```python
from build123d import *

# Parameters (mm, degrees)
F0_R     = 5
F1_DEPTH = 10
F2_R     = 3
F3_DEPTH = 7
F4_W     = 0.5
F4_H     = 1
F6_SIZE  = 1
F7_SIZE  = 1


with BuildPart() as f1:
    # F0 (on Top) → F1 (new body)
    with BuildSketch(Plane.XY):
        Circle(F0_R)
    extrude(amount=F1_DEPTH)

    # F2 (on face) → F3 (join)
    with BuildSketch(Plane.XY.offset(10)):
        Circle(F2_R)
    extrude(amount=F3_DEPTH)

    # F4 (on Front) → F5 (revolve, cut)
    with BuildSketch(Plane.XZ):
        with Locations((2.75, 10.5)):
            Rectangle(F4_W, F4_H)
    revolve(axis=Axis((0, 0, 10), (0, 0, -1)), mode=Mode.SUBTRACT)

    # F6
    f6_edges = [f1.edges().sort_by_distance(p)[0] for p in [
        (-3, 0, 17),
    ]]
    chamfer(f6_edges, length=F6_SIZE)

    # F7
    f7_edges = [f1.edges().sort_by_distance(p)[0] for p in [
        (-5, 0, 0),
    ]]
    chamfer(f7_edges, length=F7_SIZE)


solid = f1.part
```
Source: CAD feature listing. Evaluate the final solid. Frame: model axes, mm. A direction names the side the tool comes from. Round coordinates to 2 decimals unless told otherwise and drop trailing zeros. Write each loop counter-clockwise with the first axis right and the second up, starting at its lowest first coordinate (ties: lowest second). Pieces come first, ordered by that corner, then holes. Notation, with made-up numbers: M 62,73.25 L 69,73.25 A28 cw 69,100.25 Z; hole C 83,-20.75 d4. An arc over 180 degrees is marked long. Answer as a JSON object with one key per item and string values. Group by question number.
(1) First-contact query: pin 1 (6 mm diameter, centred on x = -2.5, y = 2, fed in from -Z); pin 2 (3 mm diameter, centred on y = -2, z = 10, fed in from +X); pin 3 (2 mm diameter, centred on y = -2, z = 4, fed in from +X); pin 4 (1.5 mm diameter, centred on x = -0.5, z = 13.5, fed in from +Y). Flat tips, straight axial feed; report the tip coordinate or a pass-through.
(2) Section query D-D on z = 6.25. Output: boundary loops of the cut face in (x, y).
(3) Reachability of faces 4 (the flat face through (0, 0, 0)), 5 (the cylindrical face through (-0.54, 2.44, 10.51)), 6 (the cylindrical face through (-3, 0, 13)) from +Z, -Z, +X, -X, +Y, -Y: full face, straight path, thin tool, end or side. Return the list, or none.
(4) Ray query, line 1 (X direction, y = -3, z = 2.75); line 2 (Z direction, x = 2.75, y = -2.25). Return the intervals inside material, ascending. Write a range as [from, to].
(5) Mould query, pull axis Z, two halves, no side actions, for faces 1 (the flat face through (2, -2, 11)), 2 (the flat face through (0, 0, 17)), 3 (the cylindrical face through (-1.08, -4.88, 5.44)). Classes: +Z half, -Z half, draft (parallel to the pull), parting line (faces both ways), or undercut.
(6) Section query A-A on y = 0. Output: boundary loops of the cut face in (x, z).
(7) Section query C-C on z = 12.5. Output: boundary loops of the cut face in (x, y), then the cut area to 3 significant figures.
Computed values:
{
 "1": {"pin 1": "z = 0", "pin 2": "x = 4.97", "pin 3": "x = 4.9", "pin 4": "y = 3"},
 "2": {"outline": "C 0,0 d10"},
 "3": {"face 4": "-Z, +X, -X, +Y, -Y", "face 5": "none", "face 6": "+Z"},
 "4": {"line 1": "[-4, 4]", "line 2": "[0, 10]"},
 "5": {"face 1": "undercut", "face 2": "+Z half", "face 3": "draft"},
 "6": {"outline": "M -5,1 L -4,0 L 4,0 L 5,1 L 5,10 L 2.5,10 L 2.5,11 L 3,11 L 3,16 L 2,17 L -2,17 L -3,16 L -3,11 L -2.5,11 L -2.5,10 L -5,10 Z"},
 "7": {"outline": "C 0,0 d6", "area": "28.3 mm^2"}
}
